Here's how the part is built. I have some questions about the finished solid (model axes, mm). A direction names the side the tool comes from. Round coordinates to 2 decimals unless told otherwise and drop trailing zeros. Write each loop counter-clockwise with the first axis right and the second up, starting at its lowest first coordinate (ties: lowest second). Pieces come first, ordered by that corner, then holes. Notation, with made-up numbers: M -1.5,55.25 L 14.5,55.25 A28 ccw 14.5,94.25 Z; hole C -25,-31.5 d1. An arc over 180 degrees is marked long. Use a Markdown table: item, result. Add a question column.
Autodesk Inventor part; units mm, degrees
ref_plane "Work Plane1" through (-40, 0, 0) normal (1, 0, 0) x (0, 0, -1)
ref_plane "YZ Plane" through (0, 0, 0) normal (1, 0, 0) x (0, 1, 0)
ref_plane "XZ Plane" through (0, 0, 0) normal (0, 1, 0) x (-1, 0, 0)
sketch "Sketch1" plane through (0, 0, 0) normal (0, 1, 0) x (-1, 0, 0)
  line L0 (0, 0) -> (80, 0)
  line L1 (80, 0) -> (80, -20)
  line L2 (80, -20) -> (0, -20)
  line L3 (0, -20) -> (0, 0)
  dimension "d0" = 80
  dimension "d1" = 20
extrude "Extrusion1" add sketch "Sketch1" along normal blind 70
sketch "Sketch2" plane through (0, 70, 0) normal (0, 1, 0) x (1, 0, 0)
  line L0 (0, 20) -> (-80, 20)
  line L1 (-70, 0) -> (-60, 0)
  line L2 (-60, 0) -> (-60, 20)
  line L3 (-60, 20) -> (-70, 20)
  line L4 (-70, 20) -> (-70, 0)
  line L5 (-80, 0) -> (0, 0)
  line L6 (-10, 0) -> (-20, 0)
  line L7 (-20, 0) -> (-20, 20)
  line L8 (-20, 20) -> (-10, 20)
  line L9 (-10, 20) -> (-10, 0)
  line L10 (-40, 0) -> (-40, 20)
  dimension "d4" = 10
  dimension "d5" = 10
  dimension "d6" = 40
extrude "Extrusion2" add sketch "Sketch2" along normal blind 30 contours L9 L5 L7 L0 | L2 L1 L4 L0
hole "Hole1" at (-10, 90, -10) direction (-1, 0, 0) diameter 13.5 end through all
fillet "Fillet1" radius 5 2 edges at (-20, 70, -10) (-60, 70, -10)
fillet "Fillet2" radius 10 4 edges at (-15, 100, 0) (-65, 100, 0) (-65, 100, -20) (-15, 100, -20)
sketch "Sketch3" plane through (0, 0, 0) normal (1, 0, 0) x (0, 0, -1)
  line L0 (0, 70) -> (20, 70)
  line L1 (10, 70) -> (10, 0)
  line L2 (0, 0) -> (20, 0)
  point P0 (10, 52)
  point P1 (10, 18)
  dimension "d20" = 18
  dimension "d21" = 18
hole "Hole2" at (0, 52, -10) at (0, 18, -10) direction (-1, 0, 0) diameter 11.835 depth 24 tip angle 118
ref_plane "Work Plane1" through (-40, 0, 0) normal (1, 0, 0) x (0, 0, -1)
mirror "Mirror1" about plane through (-40, 0, 0) normal (1, 0, 0) of "Hole2"
fillet "Fillet3" radius 10 2 edges at (-10, 70, -10) (-70, 70, -10)
properties part number "Profile_Middle_06" material "Aluminum 6061 T6 80 Hot Formed"
Item 1: If we mould it in two halves opening along X, with no side actions, what happens to faces 1 (the face through (-40, 70, -10)), 2 (the face through (-80, 35, -10)), 3 (the face through (-39, 34, 0)), 4 (the face through (0, 35, -10))? For each: +X half, -X half, draft (parallel to the pull), parting line (faces both ways), or undercut.
Item 2: Imagine slicing it at C-C on x = -39.5. List the corners of the cut face in (y, z) for me.
Item 3: For pin 1 Ø6 at (x, z) = (-44, -8.5) entering from +Y; pin 2 Ø9.5 at (y, z) = (52, -10) entering from +X; pin 3 Ø10.5 at (y, z) = (18, -10) entering from -X; pin 4 Ø1.5 at (x, z) = (-66, -17) entering from -Y, each with a flat end and sliding along its axis, tell me the tip position at first contact or that it passes through.
Item 4: Imagine slicing it at A-A on x = -62.5. Count the separate pieces of the cut face and the enclosed holes in it, plus the area to 3 significant figures.
Item 5: I need wall thicknesses on probe 1 along Y at (x, z) = (-18.5, -10); probe 2 along Y at (x, z) = (-60.5, -13.25); probe 3 along Y at (x, z) = (-8.5, -10). Which ranges of each line are inside material? Lowest first, please. Write a range as from..to.
Item 6: On a 3-axis mill with a long thin cutter (end or side, diameter ignored), from which of +Z, -Z, +X, -X, +Y, -Y can I reach the whole of each face in a straight line? I mean faces 5 (the face through (-67.832, 57.867, -9.23)), 6 (the face through (-70, 83, -10)), 7 (the face through (-12.168, 55.601, -5.304)), 8 (the face through (-20, 82, -10)). Say none if no direction works.
Item 7: Imagine slicing it at B-B on y = 78. List the corners of the cut face in (x, z) for me, plus the area to 3 significant figures.
The answers:
| question | item | result |
|---|---|---|
| 1 | face 1 | undercut |
| 1 | face 2 | -X half |
| 1 | face 3 | draft |
| 1 | face 4 | +X half |
| 2 | outline | M 0,-20 L 70,-20 L 70,0 L 0,0 Z |
| 3 | pin 1 | y = 70 |
| 3 | pin 2 | x = -24.7 |
| 3 | pin 3 | x = -55.6 |
| 3 | pin 4 | y = 0 |
| 4 | separate pieces | 1 |
| 4 | enclosed holes | 3 |
| 4 | area | 1,590 mm² |
| 5 | probe 1 | 0..12.08, 23.92..46.08, 57.92..83.25, 96.75..100 |
| 5 | probe 2 | 0..13.05, 22.95..47.05, 56.95..84.08, 95.92..99.46 |
| 5 | probe 3 | 0..12.08, 23.92..46.08, 57.92..74.73 |
| 6 | face 5 | -X |
| 6 | face 6 | +Z, -Z, -X, +Y |
| 6 | face 7 | +X |
| 6 | face 8 | +Z, -Z, +Y |
| 7 | outline | M -70.2,-20 L -60,-20 L -60,0 L -70.2,0 Z; M -20,-20 L -9.8,-20 L -9.8,0 L -20,0 Z |
| 7 | area | 408 mm² |
